Design review of the part shown in the three views and the two pictorial views. Dimensions are in mm from the part's minimum x, y and z. Round coordinates to 2 decimals unless told otherwise and drop trailing zeros. Write each loop counter-clockwise with the first axis right and the second up, starting at its lowest first coordinate (ties: lowest second). Pieces come first, ordered by that corner, then holes. Notation, with made-up numbers: (40.25, 33) - (52.25, 33) arc R20 ccw to (52.25, 39) - close; hole circle Ø4 at (-27.5, 44.5). An arc over 180 degrees is marked (long way). Use one line per item in the form item = value.
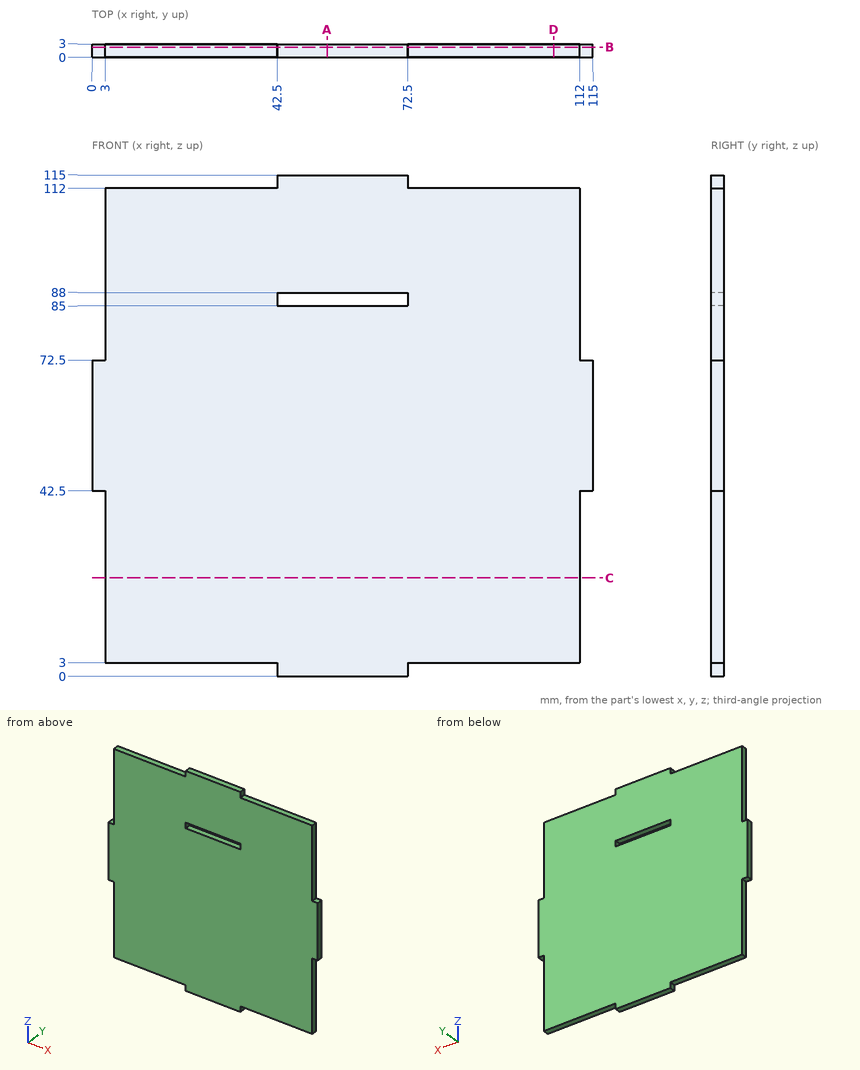
(1) Add section B-B on y = 2.3. Write out the cut boundary in (x, z), then the cut area to 3 significant figures.
Geometry results:
outline = (0, 42.5) - (3, 42.5) - (3, 3) - (42.5, 3) - (42.5, 0) - (72.5, 0) - (72.5, 3) - (112, 3) - (112, 42.5) - (115, 42.5) - (115, 72.5) - (112, 72.5) - (112, 112) - (72.5, 112) - (72.5, 115) - (42.5, 115) - (42.5, 112) - (3, 112) - (3, 72.5) - (0, 72.5) - close; hole (42.5, 85) - (72.5, 85) - (72.5, 88) - (42.5, 88) - close
area = 12,200 mm2
(2) Insertion check: P1, Ø1, axis at x = 21, y = 2, coming from the -Z side; P2, Ø0.9, axis at y = 1.5, z = 86.5, coming from the -X side; P3, Ø1.5, axis at x = 52.5, y = 1.5, coming from the -Z side; P4, Ø1.5, axis at y = 1.5, z = 1, coming from the +X side. Each pin has a flat end and moves straight along its axis. Give the tip position at first contact, or say it passes through.
Geometry results:
P1 = 3
P2 = 3
P3 = 0
P4 = 72.5
(3) Add section C-C on z = 22.5. Write out the cut boundary in (x, y).
Geometry results:
outline = (3, 0) - (112, 0) - (112, 3) - (3, 3) - close
(4) To check wall thickness, follow L1, parallel to Z at x = 71.5, y = 1.3; L2, parallel to X at y = 0.35, z = 41. State the ranges of each line that lie inside material, in increasing order.
Geometry results:
L1 = 0 to 85, 88 to 115
L2 = 3 to 112
(5) Add section D-D on x = 106. Write out the cut boundary in (y, z).
Geometry results:
outline = (0, 3) - (3, 3) - (3, 112) - (0, 112) - close
(6) Add section A-A on x = 54. Write out the cut boundary in (y, z).
Geometry results:
outline = (0, 0) - (3, 0) - (3, 85) - (0, 85) - close; (0, 88) - (3, 88) - (3, 115) - (0, 115) - close
